```python
from build123d import *

# Parameters (mm, degrees)
SKETCH1_R           = 3
BOSS_EXTRUDE1_DEPTH = 5


with BuildPart() as part:
    # Sketch1 → Boss-Extrude1 (new body)
    with BuildSketch(Plane(origin=(0, 0, 0), x_dir=(1, 0, 0), z_dir=(0, 1, 0))):
        with BuildLine():
            Line((0, 7.5), (100, 7.5))
            ThreePointArc((100, 7.5), (107.5, 0), (100, -7.5))
            Line((100, -7.5), (0, -7.5))
            ThreePointArc((0, -7.5), (-7.5, 0), (0, 7.5))
        make_face()
        with Locations((100, 0)):
            Circle(SKETCH1_R, mode=Mode.SUBTRACT)
        Circle(SKETCH1_R, mode=Mode.SUBTRACT)
    extrude(amount=BOSS_EXTRUDE1_DEPTH)


solid = part.part
```
For this review, take the finished solid that the model builds, in its own axes (mm). Give positions to 0.01 mm unless a question says otherwise; leave off trailing zeros. Loops run counter-clockwise (first coordinate to the right, second up) from the corner with the lowest first, then second, coordinate; pieces in that order, holes last. Notation, with made-up numbers: M -37.75,26.5 L 3.25,26.5 A25 ccw 3.25,48.5 Z; hole C 82.25,28.25 d5. An arc over 180 degrees is marked long. One line per item, written item: value. Start each with the question number.
Q1. For L1, parallel to X at y = 2.7, z = 0; L2, parallel to Z at x = 0, y = 3; L3, parallel to X at y = 1.3, z = 2.75, list the stretches that pass through material, from the lowest coordinate up.
Q2. Add section B-B (y = 3.55). Give the boundary of the cut face in (x, z), and give its area (3 significant figures).
Q3. Add section A-A (z = 0). Give the boundary of the cut face in (x, y).
Q4. Add section C-C (z = 5.75). Give the boundary of the cut face in (x, y).
Q5. Draft analysis for pull direction X (two halves, no side actions). For faces 1 (the face through (97, 2, 0)), 2 (the face through (51, 0, 0)), 3 (the face through (107.5, 2.46, -0.16)), state which applies: released by +X, released by -X, zero draft, split by the parting line, or undercut.
Q6. Add section D-D (z = -4.25). Give the boundary of the cut face in (x, y), and give its area (3 significant figures).
Reply:
1. L1: -7.5 to -3, 3 to 97, 103 to 107.5
1. L2: -7.5 to -3, 3 to 7.5
1. L3: -6.98 to -1.2, 1.2 to 98.8, 101.2 to 106.98
2. outline: M 0,-7.5 L 100,-7.5 A7.5 ccw 100,7.5 L 0,7.5 A7.5 ccw Z; hole C 0,0 d6; hole C 100,0 d6
2. area: 1,620 mm²
3. outline: M -7.5,0 L -3,0 L -3,5 L -7.5,5 Z; M 3,0 L 97,0 L 97,5 L 3,5 Z; M 103,0 L 107.5,0 L 107.5,5 L 103,5 Z
4. outline: M -4.82,0 L 104.82,0 L 104.82,5 L -4.82,5 Z
5. face 1: undercut
5. face 2: zero draft
5. face 3: released by +X
6. outline: M -6.18,0 L 106.18,0 L 106.18,5 L -6.18,5 Z
6. area: 562 mm²
